Read the model definition and answer for the solid it produces. Units are mm, in the model's axes. Face numbers are marked on the shaded views. A direction names the side the tool comes from. Give positions to 0.01 mm unless a question says otherwise; leave off trailing zeros. Loops run counter-clockwise (first coordinate to the right, second up) from the corner with the lowest first, then second, coordinate; pieces in that order, holes last. Notation, with made-up numbers: (-4.75, -1.5) -> (18.25, -1.5) arc R26 cw to (18.25, 14.5) -> close; hole circle Ø8 at (-3, 42.25). An arc over 180 degrees is marked (long way). Return JSON: item names as keys, results as strings. Group by question number.
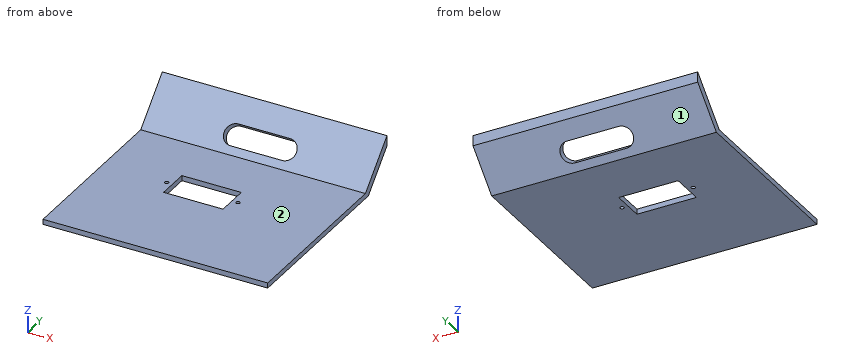
from build123d import *

# Parameters (mm, degrees)
SKETCH_1_W          = 87
SKETCH_1_H          = 70
EXTRUDE_1_DEPTH     = 2
EXTRUDE_2_DEPTH     = 87
SKETCH_6_W          = 23
SKETCH_6_H          = 12.7
CUT_EXTRUDE_1_DEPTH = 15
SKETCH_7_R          = 0.75
CUT_EXTRUDE_2_DEPTH = 15
CUT_EXTRUDE_3_DEPTH = 5


with BuildPart() as part:
    # 草图1 → 凸台-拉伸1 (new body)
    with BuildSketch(Plane.XY):
        with Locations((-41.5, -157.880838162)):
            Rectangle(SKETCH_1_W, SKETCH_1_H)
    extrude(amount=EXTRUDE_1_DEPTH)

    # 草图3 → 凸台-拉伸2 (add)
    with BuildSketch(Plane(origin=(2, 0, 0), x_dir=(0, 0, -1), z_dir=(1, 0, 0))):
        Polygon((-17, -109.880838162), (-2, -124.880838162), (0, -122.880838162), (-13, -109.880838162), align=None)
    extrude(amount=-EXTRUDE_2_DEPTH)

    # 草图6 → 切除-拉伸1 (cut)
    with BuildSketch(Plane.XY.offset(2)):
        with Locations((-46.550124355, -151.030838162)):
            Rectangle(SKETCH_6_W, SKETCH_6_H)
    extrude(amount=-CUT_EXTRUDE_1_DEPTH, mode=Mode.SUBTRACT)

    # 草图7 → 切除-拉伸2 (cut)
    with BuildSketch(Plane.XY.offset(2)):
        with Locations((-32.750124355, -151.130838162)):
            Circle(SKETCH_7_R)
        with Locations((-60.350124355, -151.130838162)):
            Circle(SKETCH_7_R)
    extrude(amount=-CUT_EXTRUDE_2_DEPTH, mode=Mode.SUBTRACT)

    # 草图8 → 切除-拉伸3 (cut)
    with BuildSketch(Plane(origin=(0, -63.440419081, 63.440419081), x_dir=(1, 0, 0), z_dir=(0, -0.707106781186556, 0.7071067811865391))):
        with BuildLine():
            Line((-51.5, -75.764432966), (-31.5, -75.764432966))
            ThreePointArc((-31.5, -75.764432966), (-27.5, -79.764432966), (-31.5, -83.764432966))
            Line((-31.5, -83.764432966), (-51.5, -83.764432966))
            ThreePointArc((-51.5, -83.764432966), (-55.5, -79.764432966), (-51.5, -75.764432966))
        make_face()
    extrude(amount=-CUT_EXTRUDE_3_DEPTH, mode=Mode.SUBTRACT)


solid = part.part
1. Straight lines are drawn through the part: line 1 (Z direction, x = -41, y = -174); line 2 (Y direction, x = -68, z = 12.75); line 3 (Y direction, x = -49, z = 14). For each, find the intervals that lie inside material, in ascending order. Write a range as from..to.
2. Section A-A on x = -11 is taken. Determine the outline of the cut face in (y, z), then the cut area to 3 significant figures.
3. Section C-C on x = -52.5 is taken. Determine the outline of the cut face in (y, z), then the cut area to 3 significant figures.
4. Section B-B on y = -181.5 is taken. Determine the outline of the cut face in (x, z), then the cut area to 3 significant figures.
5. Which of the six approach directions +Z, -Z, +X, -X, +Y, -Y give full straight-line access (tool end or side, diameter ignored) to the marked faces 1 and 2?
6. Flat-ended cylindrical pins translate along their axes: pin 1 Ø2.5 at (x, y) = (-32.75, -151.13) entering from +Z; pin 2 Ø2 at (x, y) = (-60.35, -151.13) entering from -Z; pin 3 Ø4 at (x, z) = (-55, 5.5) entering from -Y; pin 4 Ø2 at (x, z) = (-43.5, 1) entering from +Y. Find the tip coordinate at first contact, or state that the pin passes through.
Completed:
{
 "1": {"line 1": "z = 0..2", "line 2": "y = -114.13..-110.13", "line 3": "y = -112.88..-109.88"},
 "2": {"outline": "(-192.88, 0) -> (-122.88, 0) -> (-109.88, 13) -> (-109.88, 17) -> (-124.88, 2) -> (-192.88, 2) -> close", "area": "194 mm²"},
 "3": {"outline": "(-192.88, 0) -> (-157.38, 0) -> (-157.38, 2) -> (-192.88, 2) -> close; (-144.68, 0) -> (-122.88, 0) -> (-120.58, 2.3) -> (-122.58, 4.3) -> (-124.88, 2) -> (-144.68, 2) -> close; (-117.1, 9.78) -> (-115.1, 7.78) -> (-109.88, 13) -> (-109.88, 17) -> close", "area": "147 mm²"},
 "4": {"outline": "(-85, 0) -> (2, 0) -> (2, 2) -> (-85, 2) -> close", "area": "174 mm²"},
 "5": {"face 1": "-Z, +X, -X, +Y", "face 2": "+Z, +X, -X, -Y"},
 "6": {"pin 1": "stops at z = 2", "pin 2": "stops at z = 0", "pin 3": "stops at y = -123.38", "pin 4": "stops at y = -120.88"}
}
